Geometry check sheet. Reference: the model listing, model coordinates, mm. Give positions to 0.01 mm unless a question says otherwise; leave off trailing zeros. Write each loop counter-clockwise with the first axis right and the second up, starting at its lowest first coordinate (ties: lowest second). Pieces come first, ordered by that corner, then holes. Notation, with made-up numbers: M 32.25,0 L 55.25,0 A29 ccw 55.25,27 Z; hole C 75.5,42 d10. An arc over 180 degrees is marked long. Write each question's results on one line, items separated by ' | '.
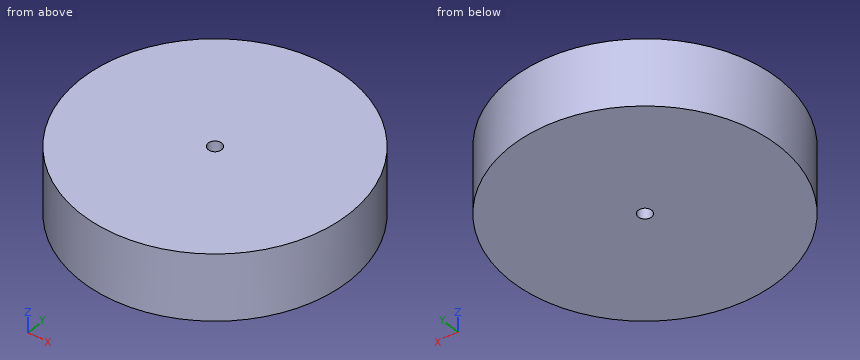
Autodesk Fusion 360 part; units mm, degrees
sketch "Sketch2" plane through (0, 0, 0) normal (0, 0, 1) x (1, 0, 0)
  circle A0 centre (0, 0) radius 20
  circle A1 centre (0, 0) radius 1
  dimension "d22" = 40
extrude "Extrude1" add sketch "Sketch2" along normal blind 10 makes body 1
copy_body "Body->Comp1" bodies 1 removing the originals makes body 2 in component "Component"
component "Component" placed x (1, 0, 0) y (0, 1, 0) z (0, 0, 1) at (0, 0, 0)
Q1. Section check C-C (z = 9.25). Enter the section's corners in (x, y).
Answer key:
outline: C 0,0 d40; hole C 0,0 d2
Q2. Depth check by flat-ended pin: P1, Ø1.6, axis at x = 0, y = 0, coming from the +Z side (1 decimal); P2, Ø2, axis at y = -12.5, z = 5.5, coming from the -X side; P3, Ø1, axis at x = 5.5, z = 2, coming from the +Y side. Enter the tip coordinate at first touch or a pass-through.
Answer key:
P1: passes through | P2: stops at x = -16.36 | P3: stops at y = 19.36
Q3. Material ranges on probe 1 along Y at (x, z) = (0, 3.5); probe 2 along X at (y, z) = (-0.5, 3.75); probe 3 along Y at (x, z) = (-14, 5.75), recorded low to high. Write a range as [from, to].
Answer key:
probe 1: y = [-20, -1], [1, 20] | probe 2: x = [-19.99, -0.87], [0.87, 19.99] | probe 3: y = [-14.28, 14.28]
Q4. Section check D-D (x = -12). Enter the section's corners in (y, z), then the cut area to 3 significant figures.
Answer key:
outline: M -16,0 L 16,0 L 16,10 L -16,10 Z | area: 320 mm2
Q5. Section check A-A (y = 0). Enter the section's corners in (x, z), then the cut area to 3 significant figures.
Answer key:
outline: M -20,0 L -1,0 L -1,10 L -20,10 Z; M 1,0 L 20,0 L 20,10 L 1,10 Z | area: 380 mm2
